Autodesk Inventor part; units mm, degrees
ref_plane "РабПлоскость1" through (0, 0, 0) normal (0, 0, 1) x (1, 0, 0)
ref_plane "YZ Plane" through (0, 0, 0) normal (1, 0, 0) x (0, 1, 0)
ref_plane "XZ Plane" through (0, 0, 0) normal (0, 1, 0) x (-1, 0, 0)
sketch "Эскиз1" plane through (0, 0, 0) normal (0, 0, 1) x (1, 0, 0)
  line L0 (-15, 5) -> (15, 5)
  line L1 (15, 5) -> (15, -5)
  line L2 (15, -5) -> (-15, -5)
  line L3 (-15, -5) -> (-15, 5)
  point P0 (0, 0)
  point P1 (0, 5)
  point P2 (15, 0)
  dimension "d0" = 30
  dimension "d1" = 10
extrude "Выдавливание1" add sketch "Эскиз1" against normal blind 10
sketch "Эскиз2" plane through (0, 0, 0) normal (0, 0, 1) x (1, 0, 0)
  line L0 (-7.5853, 4.0771) -> (10.7261, 4.0771) construction
  line L1 (10.7261, 4.0771) -> (10.7261, -0.5016) construction
  line L2 (10.7261, -0.5016) -> (-7.5853, -0.5016) construction
  line L3 (-7.5853, -0.5016) -> (-7.5853, 4.0771) construction
  point P0 (0, 0)
ref_plane "РабПлоскость1" through (0, 0, 0) normal (0, 0, 1) x (1, 0, 0)
sketch "Эскиз3" plane through (0, 0, 0) normal (0, 0, 1) x (1, 0, 0)
  circle A0 centre (-7.775, -2.4968) radius 0.5
  circle A1 centre (8.8496, -2.4968) radius 0.5
  point P0 (0, 0)
  dimension "d5" = 1
  dimension "d6" = 1
extrude "Выдавливание2" add sketch "Эскиз3" along normal blind 0.3
sketch "Эскиз4" plane through (0, 0, 0) normal (0, 0, 1) x (1, 0, 0)
  circle A0 centre (-7.775, -2.4968) radius 0.5
  circle A1 centre (-7.775, -2.4968) radius 0.1
  circle A2 centre (8.8496, -2.4968) radius 0.5
  circle A3 centre (8.8496, -2.4968) radius 0.1
  point P0 (0, 0)
  dimension "d9" = 0.2
  dimension "d10" = 0.2
extrude "Выдавливание3" add sketch "Эскиз4" along normal blind 0.4 contours A1 | A3
properties part number "lock-in"
Geometry: final body of the model. Coordinates: model frame, mm. Round coordinates to 2 decimals unless told otherwise and drop trailing zeros. Order: outer loops, then holes, each group sorted by start corner. A loop starts at its lowest first (then second) coordinate and runs counter-clockwise, first axis right, second up. Notation, with made-up numbers: (42, 88) - (65, 88) arc R17 cw to (65, 117) - close; hole circle Ø11 at (2, -12). An arc over 180 degrees is marked (long way). Use CSV: the item, a comma, the result in double quotes. Start each with the question number.
Q1. First-contact query: pin 1 (1.5 mm diameter, centred on x = 8, y = 3.5, fed in from +Z); pin 2 (0.8 mm diameter, centred on x = -8, y = -2, fed in from +Z). Flat tips, straight axial feed; report the tip coordinate or a pass-through.
Q2. Section query B-B (x = 6). Return loops of the section in (y, z).
Q3. Section query A-A (y = 4.5). Return loops of the section in (x, z), and give its area (3 significant figures).
Q4. Material intervals for line 1 along Z through (x, y) = (1.25, -3), sorted ascending. Write a range as from..to.
Result set:
1,pin 1,"stops at z = 0"
1,pin 2,"stops at z = 0.3"
2,outline,"(-5, -10) - (5, -10) - (5, 0) - (-5, 0) - close"
3,outline,"(-15, -10) - (15, -10) - (15, 0) - (-15, 0) - close"
3,area,"300 mm2"
4,line 1,"z = -10..0"
